from build123d import *

# Parameters (mm, degrees)
SKETCH_1_W             = 130
SKETCH_1_H             = 90
SKETCH_1_W_2           = 71.7
SKETCH_1_H_2           = 38.9
EXTRUDE_399_DEPTH      = 4
CUT_EXTRUDE_706_DEPTH  = 1.2
SKETCH_3_W             = 5.8
SKETCH_3_H             = 13.4
USB_DEPTH              = 80.158069709
SKETCH_4_W             = 4.4
SKETCH_4_H             = 12
CUT_EXTRUDE_1602_DEPTH = 80.106510478
USB_2_DEPTH            = 0.5
SKETCH_8_W             = 1.5
SKETCH_8_H             = 18.480447519
USB_3_DEPTH            = 1.2
XT60_DEPTH             = 80.158069709
SKETCH_9_R             = 1.55
CUT_EXTRUDE_6_DEPTH    = 80.158069709


with BuildPart() as part:
    # Эскиз1 → Extrude 399 (new body)
    with BuildSketch(Plane(origin=(0, 0, 0), x_dir=(1, 0, 0), z_dir=(0, 1, 0))):
        Rectangle(SKETCH_1_W, SKETCH_1_H)
        with Locations((15.15, 11.55)):
            Rectangle(SKETCH_1_W_2, SKETCH_1_H_2, mode=Mode.SUBTRACT)
    extrude(amount=EXTRUDE_399_DEPTH)

    # Эскиз2 → Cut-Extrude 706 (cut)
    with BuildSketch(Plane(origin=(0, 4, 0), x_dir=(1, 0, 0), z_dir=(0, 1, 0))):
        with BuildLine():
            Line((-23.6, 33.05), (53.9, 33.05))
            ThreePointArc((53.9, 33.05), (54.607106781, 32.757106781), (54.9, 32.05))
            Line((54.9, 32.05), (54.9, -8.95))
            ThreePointArc((54.9, -8.95), (54.607106781, -9.657106781), (53.9, -9.95))
            Line((53.9, -9.95), (-23.6, -9.95))
            ThreePointArc((-23.6, -9.95), (-24.307106781, -9.657106781), (-24.6, -8.95))
            Line((-24.6, -8.95), (-24.6, 32.05))
            ThreePointArc((-24.6, 32.05), (-24.307106781, 32.757106781), (-23.6, 33.05))
        make_face()
    extrude(amount=-CUT_EXTRUDE_706_DEPTH, mode=Mode.SUBTRACT)

    # Эскиз3 → USB (cut, through all)
    with BuildSketch(Plane(origin=(0, 4, 0), x_dir=(1, 0, 0), z_dir=(0, 1, 0))):
        with BuildLine():
            Line((-50.1, -4.75), (-50.1, 8.65))
            Line((-50.1, 8.65), (-43.7, 8.65))
            Line((-43.7, 8.65), (-43.7, 11.1))
            Line((-43.7, 11.1), (-42.4, 11.1))
            Line((-42.4, 11.1), (-42.4, 6.35))
            Line((-42.4, 6.35), (-39.6, 6.35))
            ThreePointArc((-39.6, 6.35), (-39.246446609, 6.203553391), (-39.1, 5.85))
            Line((-39.1, 5.85), (-39.1, -1.95))
            ThreePointArc((-39.1, -1.95), (-39.246446609, -2.303553391), (-39.6, -2.45))
            Line((-39.6, -2.45), (-42.5, -2.45))
            Line((-42.5, -2.45), (-42.5, -7.2))
            Line((-42.5, -7.2), (-43.8, -7.2))
            Line((-43.8, -7.2), (-43.8, -4.75))
            Line((-43.8, -4.75), (-50.1, -4.75))
        make_face()
        with Locations((-44.6, 25.8)):
            Rectangle(SKETCH_3_W, SKETCH_3_H)
    extrude(amount=-USB_DEPTH, mode=Mode.SUBTRACT)

    # Эскиз4 → Cut-Extrude 1602 (cut, through all)
    with BuildSketch(Plane(origin=(0, 2.8, 0), x_dir=(1, 0, 0), z_dir=(0, 1, 0))):
        with Locations((-20.7, 11.55)):
            Rectangle(SKETCH_4_W, SKETCH_4_H)
        with Locations((50.8, 11.55)):
            Rectangle(SKETCH_4_W, SKETCH_4_H)
    extrude(amount=-CUT_EXTRUDE_1602_DEPTH, mode=Mode.SUBTRACT)

    # Эскиз7 → USB 2 (cut)
    with BuildSketch(Plane(origin=(0, 4, 0), x_dir=(1, 0, 0), z_dir=(0, 1, 0))):
        with BuildLine():
            Line((-47.55, 33.05), (-41.65, 33.05))
            ThreePointArc((-41.65, 33.05), (-41.296446609, 32.903553391), (-41.15, 32.55))
            Line((-41.15, 32.55), (-41.15, 19.05))
            ThreePointArc((-41.15, 19.05), (-41.296446609, 18.696446609), (-41.65, 18.55))
            Line((-41.65, 18.55), (-47.55, 18.55))
            ThreePointArc((-47.55, 18.55), (-47.903553391, 18.696446609), (-48.05, 19.05))
            Line((-48.05, 19.05), (-48.05, 32.55))
            ThreePointArc((-48.05, 32.55), (-47.903553391, 32.903553391), (-47.55, 33.05))
        make_face()
    extrude(amount=-USB_2_DEPTH, mode=Mode.SUBTRACT)

    # Эскиз8 → USB 3 (add)
    with BuildSketch(Plane(origin=(0, 4, 0), x_dir=(1, 0, 0), z_dir=(0, 1, 0))):
        with Locations((-43.069744148, 1.932070249)):
            Rectangle(SKETCH_8_W, SKETCH_8_H)
    extrude(amount=-USB_3_DEPTH)

    # Эскиз5 → XT60 (cut, through all)
    with BuildSketch(Plane(origin=(0, 4, 0), x_dir=(1, 0, 0), z_dir=(0, 1, 0))):
        Polygon((-48.468705951, -32), (-40.468705951, -32), (-40.468705951, -18.8), (-42.951848706, -16.3), (-45.985563195, -16.3), (-48.468705951, -18.8), align=None)
    extrude(amount=-XT60_DEPTH, mode=Mode.SUBTRACT)

    # Эскиз9 → Вырез-Вытянуть6 (cut, through all)
    with BuildSketch(Plane(origin=(0, 4, 0), x_dir=(1, 0, 0), z_dir=(0, 1, 0))):
        with Locations(Location((-58, 38, 0), (0, 0, 270))):
            Circle(SKETCH_9_R)
        with Locations(Location((58, 38, 0), (0, 0, 270))):
            Circle(SKETCH_9_R)
        with Locations(Location((-58, -38, 0), (0, 0, 270))):
            Circle(SKETCH_9_R)
        with Locations(Location((58, -38, 0), (0, 0, 270))):
            Circle(SKETCH_9_R)
    extrude(amount=-CUT_EXTRUDE_6_DEPTH, mode=Mode.SUBTRACT)


solid = part.part
Build history of the part. All positions in model axes, mm. A direction names the side the tool comes from. Coordinates: 2 decimals unless noted, no trailing zeros. Write each loop counter-clockwise with the first axis right and the second up, starting at its lowest first coordinate (ties: lowest second). Pieces come first, ordered by that corner, then holes.
(1) Drill centre lines: line 1 (X direction, y = 2.25, z = 38); line 2 (X direction, y = 3.4, z = -23.5); line 3 (Z direction, x = 43, y = 2.2). Where is each one in solid material? Low to high.
(2) Cut at A-A on z = 38. List the corners of the cut face in (x, y).
(3) Cut at D-D on y = 2.15. State how many separate pieces and enclosed holes the cut face has, and give its area (3 significant figures).
(4) Mould opens along Z. For faces 1 (the flat face through (-41.5, 3.5, -26.4)), 2 (the flat face through (15, 1, -31)), 3 (the flat face through (-1, 0, 9)), 4 (the flat face through (-1, 2, -45)) say: pulls with the +Z half, pulls with the -Z half, needs draft (parallel to the pull), parting line crosses it, or undercut.
(5) 3-axis set-ups, long thin cutter, end or side, ignore diameter. For faces 5 (the flat face through (18, 2.8, 9)), 6 (the flat face through (-43.8, 1, 6)), 7 (the flat face through (-41.7, 2, -26)), 8 (the flat face through (-65, 2, 1)): which of +Z, -Z, +X, -X, +Y, -Y reach the whole face in a straight line?
(6) Cut at C-C on x = -58. List the corners of the cut face in (y, z), and give its area (3 significant figures).
(7) Pin check, flat tip, straight feed: pin 1 Ø1.2 at (x, z) = (-43, 1.5) entering from -Y. Stop position of the tip, or through.
(8) Cut at B-B on x = 28. List the corners of the cut face in (y, z).
Working result:
1. line 1: x = -65 to -59.55, -56.45 to 56.45, 59.55 to 65
1. line 2: x = -65 to -47.5, -41.7 to -24.6, 54.9 to 65
1. line 3: z = -45 to -31, 7.9 to 45
2. outline: (-65, 0) - (-59.55, 0) - (-59.55, 4) - (-65, 4) - close; (-56.45, 0) - (56.45, 0) - (56.45, 4) - (-56.45, 4) - close; (59.55, 0) - (65, 0) - (65, 4) - (59.55, 4) - close
3. separate pieces: 1
3. enclosed holes: 8
3. area: 8,490 mm2
4. face 1: undercut
4. face 2: undercut
4. face 3: needs draft
4. face 4: pulls with the -Z half
5. face 5: +Y
5. face 6: -Y
5. face 7: +Y, -Y
5. face 8: +Z, -Z, -X, +Y, -Y
6. outline: (0, -45) - (4, -45) - (4, -39.55) - (0, -39.55) - close; (0, -36.45) - (4, -36.45) - (4, 36.45) - (0, 36.45) - close; (0, 39.55) - (4, 39.55) - (4, 45) - (0, 45) - close
6. area: 335 mm2
7. pin 1: stops at y = 2.8
8. outline: (0, -45) - (4, -45) - (4, -33.05) - (2.8, -33.05) - (2.8, -31) - (0, -31) - close; (0, 7.9) - (2.8, 7.9) - (2.8, 9.95) - (4, 9.95) - (4, 45) - (0, 45) - close
